Geometry: final body of the model. Coordinates: model frame, mm. A direction names the side the tool comes from. Give positions to 0.01 mm unless a question says otherwise; leave off trailing zeros. Loops run counter-clockwise (first coordinate to the right, second up) from the corner with the lowest first, then second, coordinate; pieces in that order, holes last.
1. Access query for faces 4 (the face through (84, -26, 1)), 5 (the face through (-84, -26, 1)), 6 (the face through (-37, 26, 1)), 7 (the face through (-84, 26, 1)), 8 (the face through (36, -26, 1)). Directions: +Z, -Z, +X, -X, +Y, -Y. A direction counts if a zero-diameter tool reaches every point of the face in a straight line with its end or side. Return the directions, or none.
2. Section A-A, the plane x = 14.3. Output: boundary loops of the cut face in (y, z), then the cut area to 3 significant figures.
3. First-contact query: P1, Ø0.8, axis at y = -27, z = 2, coming from the +X side; P2, Ø0.8, axis at y = 27.5, z = 1.5, coming from the -X side; P3, Ø0.9, axis at x = -83.5, z = 1, coming from the -Y side. Flat tips, straight axial feed; report the tip coordinate or a pass-through.
4. Section B-B, the plane x = 55.5. Output: boundary loops of the cut face in (y, z).
5. Material intervals for line 1 along X through (y, z) = (14, 2.5); line 2 along Y through (x, z) = (-11.5, 1.25); line 3 along X through (y, z) = (18, 1.85), sorted ascending.
6. Draft query along X for faces 1 (the face through (-86, 0, 1)), 2 (the face through (36, 26, 1)), 3 (the face through (84, 26, 1)). Return one class per face: +X half, -X half, draft (parallel to the pull), parting line (faces both ways), or undercut.
Autodesk Inventor part; units mm, degrees
ref_plane "Plan YZ" through (0, 0, 0) normal (1, 0, 0) x (0, 1, 0)
ref_plane "Plan XZ" through (0, 0, 0) normal (0, 1, 0) x (-1, 0, 0)
ref_plane "Plan XY" through (0, 0, 0) normal (0, 0, 1) x (1, 0, 0)
sketch "Esquisse12" plane through (0, 0, 0) normal (0, 0, 1) x (1, 0, 0)
  line L0 (-86, -26) -> (-86, 26)
  line L1 (-86, 26) -> (-81, 26)
  line L2 (-81, 26) -> (-81, 29)
  line L3 (-81, 29) -> (-66, 29)
  line L4 (-66, 29) -> (-66, 26)
  line L5 (7.5, 26) -> (7.5, 29)
  line L6 (7.5, 29) -> (-7.5, 29)
  line L7 (-7.5, 29) -> (-7.5, 26)
  line L8 (66, 26) -> (66, 29)
  line L9 (66, 29) -> (81, 29)
  line L10 (81, 29) -> (81, 26)
  line L11 (81, 26) -> (86, 26)
  line L12 (86, 26) -> (86, -26)
  line L13 (86, -26) -> (81, -26)
  line L14 (81, -26) -> (81, -29)
  line L15 (81, -29) -> (66, -29)
  line L16 (66, -29) -> (66, -26)
  line L17 (-7.5, -26) -> (-7.5, -29)
  line L18 (7.5, -29) -> (7.5, -26)
  line L19 (-66, -26) -> (-66, -29)
  line L20 (-81, -29) -> (-81, -26)
  line L21 (-86, -26) -> (-81, -26)
  line L22 (-81, -29) -> (-66, -29)
  line L23 (7.5, -29) -> (-7.5, -29)
  line L24 (-66, 26) -> (-7.5, 26)
  line L25 (7.5, 26) -> (66, 26)
  line L26 (7.5, -26) -> (66, -26)
  line L27 (-7.5, -26) -> (-66, -26)
  line L28 (-120.4, 0) -> (120.4, 0) construction
  line L29 (0, -40.6) -> (0, 40.6) construction
  point P0 (0, 0)
  dimension "d86" = 52
  dimension "d87" = 3
  dimension "d88" = 5
  dimension "d90" = 15
  dimension "d112" = 172
extrude "Extrusion5" add sketch "Esquisse12" along normal blind 3
sketch "Esquisse13" plane through (0, 0, 3) normal (0, 0, 1) x (1, 0, 0)
  point P0 (0, 0)
  point P1 (-81, 26)
  point P2 (-66, 26)
  point P3 (-81, -26)
  point P4 (-66, -26)
  point P5 (-7.5, -26)
  point P6 (7.5, -26)
  point P7 (66, -26)
  point P8 (81, -26)
  point P9 (81, 26)
  point P10 (66, 26)
  point P11 (-7.5, 26)
  point P12 (7.5, 26)
hole "Perçage6" at (-81, 26, 3) at (-66, 26, 3) at (-81, -26, 3) at (-66, -26, 3) at (-7.5, -26, 3) at (7.5, -26, 3) at (66, -26, 3) at (81, -26, 3) at (81, 26, 3) at (66, 26, 3) at (-7.5, 26, 3) at (7.5, 26, 3) direction (0, 0, -1) diameter 1 end through all
chamfer "Chanfrein3" distance 1 angle 45 12 edges at (-81, 29, 1.5) (-66, 29, 1.5) (-7.5, 29, 1.5) (7.5, 29, 1.5) (66, 29, 1.5) (81, 29, 1.5) (-81, -29, 1.5) (-66, -29, 1.5) (-7.5, -29, 1.5) (7.5, -29, 1.5) (66, -29, 1.5) (81, -29, 1.5)
sketch "Esquisse14" plane through (0, 0, 3) normal (0, 0, 1) x (1, 0, 0)
  circle A0 centre (14.3, 13.8) radius 5
  line L0 (-86, -26) -> (-86, 26)
  line L1 (65.5, -26) -> (8, -26)
  point P0 (0, 0)
  dimension "d107" = 100.3
  dimension "d108" = 39.8
  dimension "d109" = 10
extrude "Extrusion6" cut sketch "Esquisse14" against normal through all
properties part number "P1704_203" material "Plastique PMMA"
Answers below:
1. face 4: +Z, -Z, +X, -Y
1. face 5: +Z, -Z, -X, -Y
1. face 6: +Z, -Z, +Y
1. face 7: +Z, -Z, -X, +Y
1. face 8: +Z, -Z, -Y
2. outline: (-26, 0) - (8.8, 0) - (8.8, 3) - (-26, 3) - close; (18.8, 0) - (26, 0) - (26, 3) - (18.8, 3) - close
2. area: 126 mm2
3. P1: stops at x = 81
3. P2: stops at x = -81
3. P3: stops at y = -26
4. outline: (-26, 0) - (26, 0) - (26, 3) - (-26, 3) - close
5. line 1: x = -86 to 9.3, 19.3 to 86
5. line 2: y = -26 to 26
5. line 3: x = -86 to 11.59, 17.01 to 86
6. face 1: -X half
6. face 2: undercut
6. face 3: draft
